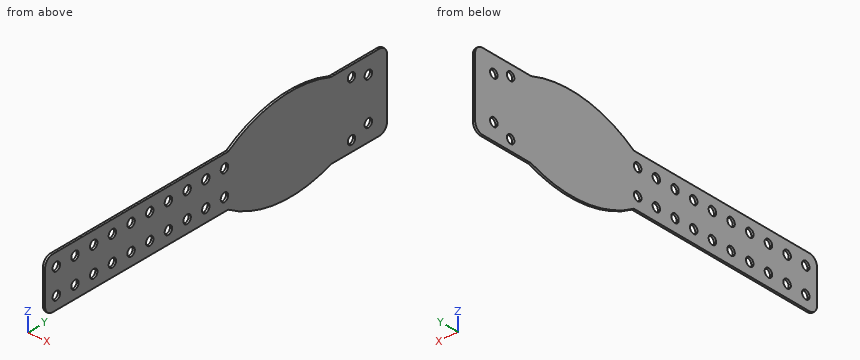
from build123d import *

# Parameters (mm, degrees)
BOSS_EXTRUDE1_DEPTH      = 1
F_4_0_4_DIAMETER_HOLE3_D = 4
F_4_0_4_DIAMETER_HOLE2_D = 4
F_4_0_4_DIAMETER_HOLE1_D = 4
LPATTERN1_COUNT          = 10
LPATTERN1_PITCH          = 10
FILLET1_R                = 4


with BuildPart() as part:
    # Sketch1 → Boss-Extrude1 (new body)
    with BuildSketch(Plane(origin=(0, 0, 0), x_dir=(0, 0, -1), z_dir=(1, 0, 0))):
        with BuildLine():
            Line((12, -183), (12, -85))
            ThreePointArc((12, -85), (21.475099597, -58.206374501), (18, -30))
            Line((18, -30), (18, 0))
            Line((18, 0), (-18, 0))
            Line((-18, 0), (-18, -30))
            ThreePointArc((-18, -30), (-21.475099597, -58.206374501), (-12, -85))
            Line((-12, -85), (-12, -183))
            Line((-12, -183), (12, -183))
        make_face()
    extrude(amount=BOSS_EXTRUDE1_DEPTH)

    # Ø4.0 (4) Diameter Hole3 (through all)
    with Locations(Plane.ZY):
        with Locations((10, -10), (-10, -10)):
            Hole(F_4_0_4_DIAMETER_HOLE3_D / 2)

    # Ø4.0 (4) Diameter Hole2 (through all)
    with Locations(Plane.ZY):
        with Locations((-13, -19), (13, -19)):
            Hole(F_4_0_4_DIAMETER_HOLE2_D / 2)

    # Ø4.0 (4) Diameter Hole1 (through all)
    with Locations(Plane(origin=(1, 0, 0), x_dir=(0, 0, -1), z_dir=(1, 0, 0))):
        with Locations((-6, -177), (6, -177)):
            f_4_0_4_diameter_hole1 = Hole(F_4_0_4_DIAMETER_HOLE1_D / 2)

    # LPattern1: Ø4.0 (4) Diameter Hole1 ×10
    with Locations(*[(0, i * LPATTERN1_PITCH, 0) for i in range(1, LPATTERN1_COUNT)]):
        add(f_4_0_4_diameter_hole1, mode=Mode.SUBTRACT)

    # Fillet1
    fillet1_edges = [part.edges().sort_by_distance(p)[0] for p in [
        (0.5, 0, 18),
        (0.5, 0, -18),
        (0.5, -183, -12),
        (0.5, -183, 12),
    ]]
    fillet(fillet1_edges, radius=FILLET1_R)


solid = part.part
Can you work these out from the model? Positions are in its coordinate system, mm. Give positions to 0.01 mm unless a question says otherwise; leave off trailing zeros. Loops run counter-clockwise (first coordinate to the right, second up) from the corner with the lowest first, then second, coordinate; pieces in that order, holes last. Notation, with made-up numbers: (-11.5, 26) -> (46.5, 26) arc R15 ccw to (46.5, 43) -> close; hole circle Ø5 at (26, -6). An arc over 180 degrees is marked (long way). Write item = value, one per line.
1) Will these pins go through, and if not, where does the flat tip stop? pin 1 (0.5 mm diameter, centred on x = 0.5, y = -119.5, fed in from +Z); pin 2 (2.5 mm diameter, centred on y = -107, z = 6, fed in from -X); pin 3 (3 mm diameter, centred on y = -47, z = 7, fed in from -X).
Check result:
pin_1 = 12
pin_2 = through
pin_3 = 0
2) Suppose I cut it at C-C on x = 0.2. Give the number of separate pieces and of enclosed holes in the cut face, then the cut area to 3 significant figures.
Check result:
separate_pieces = 1
enclosed_holes = 24
area = 5,250 mm2
3) I need wall thicknesses on L1, parallel to Z at x = 0.65, y = -177; L2, parallel to Z at x = 0.65, y = -122.5; L3, parallel to Z at x = 0.6, y = -108. Which ranges of each line are inside material? Lowest first, please. Write a range as from..to.
Check result:
L1 = -12..-8, -4..4, 8..12
L2 = -12..12
L3 = -12..-7.73, -4.27..4.27, 7.73..12
4) Suppose I cut it at A-A on y = -10. Write out the boundary of the cut face in (x, z).
Check result:
outline = (0, -18) -> (1, -18) -> (1, -12) -> (0, -12) -> close; (0, -8) -> (1, -8) -> (1, 8) -> (0, 8) -> close; (0, 12) -> (1, 12) -> (1, 18) -> (0, 18) -> close
5) Suppose I cut it at B-B on y = -117. Write out the boundary of the cut face in (x, z).
Check result:
outline = (0, -12) -> (1, -12) -> (1, -8) -> (0, -8) -> close; (0, -4) -> (1, -4) -> (1, 4) -> (0, 4) -> close; (0, 8) -> (1, 8) -> (1, 12) -> (0, 12) -> close
6) Suppose I cut it at D-D on y = -151. Write out the boundary of the cut face in (x, z).
Check result:
outline = (0, -12) -> (1, -12) -> (1, 12) -> (0, 12) -> close
